Source: CAD feature listing. Evaluate the final solid. Frame: model axes, mm. Face numbers are marked on the shaded views. A direction names the side the tool comes from. Give positions to 0.01 mm unless a question says otherwise; leave off trailing zeros. Order: outer loops, then holes, each group sorted by start corner. A loop starts at its lowest first (then second) coordinate and runs counter-clockwise, first axis right, second up.
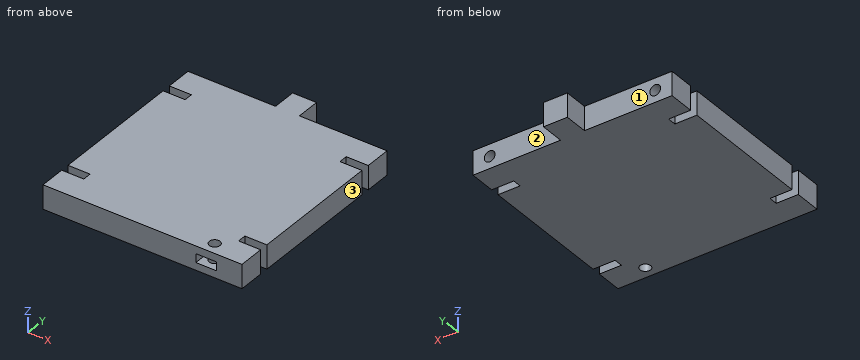
Autodesk Inventor part; units mm, degrees
ref_plane "YZ Plane" through (0, 0, 0) normal (1, 0, 0) x (0, 1, 0)
ref_plane "XZ Plane" through (0, 0, 0) normal (0, 1, 0) x (-1, 0, 0)
ref_plane "XY Plane" through (0, 0, 0) normal (0, 0, 1) x (1, 0, 0)
sketch "스케치1" plane through (0, 0, 0) normal (0, 0, 1) x (1, 0, 0)
  line L0 (0, 0) -> (50, 0)
  line L1 (50, 0) -> (50, 25)
  line L2 (0, 25) -> (50, 25)
  line L3 (0, 0) -> (0, 25)
  line L4 (8.4, 0) -> (0, 0)
  line L5 (0, 0) -> (0, -16)
  line L6 (50, -16) -> (0, -16)
  line L7 (50, 0) -> (50, -16)
  line L8 (50, 0) -> (41.6, 0)
  line L9 (41.6, 0) -> (41.6, -10)
  line L10 (41.6, -10) -> (8.4, -10)
  line L11 (8.4, 0) -> (8.4, -10)
  line L12 (0, 25) -> (50, 25)
  line L13 (50, 25) -> (50, 35)
  line L14 (50, 35) -> (0, 35)
  line L15 (0, 35) -> (0, 25)
  line L16 (0, -16) -> (50, -16)
  line L17 (50, -16) -> (50, 35)
  line L18 (50, 35) -> (0, 35)
  line L19 (0, 35) -> (0, -16)
  dimension "d0" = 10
extrude "돌출1" add sketch "스케치1" along normal blind 6
sketch "스케치2" plane through (0, 0, 6) normal (0, 0, 1) x (1, 0, 0)
  circle A0 centre (41, -13) radius 1.35
  point P0 (0, 0)
extrude "돌출2" cut sketch "스케치2" against normal up to next
sketch "스케치3" plane through (0, 35, 0) normal (0, 1, 0) x (1, 0, 0)
  line L0 (50, 0) -> (0, 0)
  line L1 (28, -6) -> (50, -6)
  line L2 (39, -6) -> (25, 0)
  line L3 (39, -6) -> (22, -6)
  line L4 (22, -6) -> (22, 0)
  line L5 (22, 0) -> (39, 0)
  line L6 (39, 0) -> (39, -6)
  line L7 (39, 0) -> (28, 0)
  line L8 (28, 0) -> (28, -6)
  line L9 (28, -6) -> (39, -6)
  line L10 (39, -6) -> (39, 0)
  point P0 (22, -6)
extrude "돌출3" add sketch "스케치3" along normal blind 6 contours L8 L2 L0 | L2 L8 L3 L4 L0
sketch "스케치4" plane through (50, 35, 6) normal (0, 1, 0) x (1, 0, 0)
  circle A0 centre (-4.2, 79) radius 1.35
  circle A1 centre (-4.2, 3) radius 1.35
  circle A2 centre (-45.8, 79) radius 1.35
  circle A3 centre (-45.8, 3) radius 1.35
  circle A4 centre (-4.2, 71.8) radius 1.6
  circle A5 centre (-45.8, 71.8) radius 1.6
  circle A6 centre (-4.2, 10.2) radius 1.6
  circle A7 centre (-45.8, 10.2) radius 1.6
  line L0 (-50, 0) -> (-28, 0)
  line L1 (-28, 0) -> (-28, 6)
  line L2 (-28, 6) -> (-22, 6)
  line L3 (-22, 6) -> (-22, 0)
  line L4 (-22, 0) -> (0, 0)
  line L5 (0, 0) -> (0, 82)
  line L6 (0, 82) -> (-50, 82)
  line L7 (-50, 82) -> (-50, 0)
  point P0 (-50, 6)
extrude "돌출4" cut sketch "스케치4" against normal blind 6 contours A1 | A3
sketch "스케치6" plane through (0, 0, 6) normal (0, 0, 1) x (1, 0, 0)
  line L0 (47.05, 26.225) -> (47.05, 40.9)
  line L1 (47.05, 31.225) -> (47.05, 40.9)
  line L2 (47.05, 26.225) -> (49.65, 26.225)
  line L3 (50, -16) -> (50, 35)
  line L4 (47.05, 26.225) -> (44.45, 26.225)
  line L5 (44.45, 26.225) -> (44.45, 28.425)
  line L6 (44.45, 28.425) -> (49.65, 28.425)
  line L7 (49.65, 28.425) -> (49.65, 26.225)
  line L8 (28, 41) -> (22, 41)
  line L9 (25, 41) -> (25, 38)
  line L10 (2.95, 26.225) -> (0.35, 26.225)
  line L11 (2.95, 26.225) -> (5.55, 26.225)
  line L12 (5.55, 26.225) -> (5.55, 28.425)
  line L13 (5.55, 28.425) -> (0.35, 28.425)
  line L14 (0.35, 28.425) -> (0.35, 26.225)
  line L15 (0, 35) -> (0, -16)
  line L16 (0.35, 26.225) -> (0, 26.225)
  line L17 (0, 26.225) -> (0, 28.425)
  line L18 (0, 28.425) -> (0.35, 28.425)
  line L19 (0.35, 28.425) -> (0.35, 26.225)
  line L20 (49.65, 28.425) -> (50, 28.425)
  line L21 (50, 28.425) -> (50, 26.225)
  line L22 (50, 26.225) -> (49.65, 26.225)
  line L23 (49.65, 26.225) -> (49.65, 28.425)
  line L24 (0, 9.5) -> (2.95, 9.5)
  line L25 (47.05, -7.225) -> (49.65, -7.225)
  line L26 (47.05, -7.225) -> (44.45, -7.225)
  line L27 (44.45, -7.225) -> (44.45, -9.425)
  line L28 (44.45, -9.425) -> (49.65, -9.425)
  line L29 (49.65, -9.425) -> (49.65, -7.225)
  line L30 (2.95, -7.225) -> (0.35, -7.225)
  line L31 (2.95, -7.225) -> (5.55, -7.225)
  line L32 (5.55, -7.225) -> (5.55, -9.425)
  line L33 (5.55, -9.425) -> (0.35, -9.425)
  line L34 (0.35, -9.425) -> (0.35, -7.225)
  line L35 (0.35, -7.225) -> (0, -7.225)
  line L36 (0, -7.225) -> (0, -9.425)
  line L37 (0, -9.425) -> (0.35, -9.425)
  line L38 (0.35, -9.425) -> (0.35, -7.225)
  line L39 (49.65, -9.425) -> (50, -9.425)
  line L40 (50, -9.425) -> (50, -7.225)
  line L41 (50, -7.225) -> (49.65, -7.225)
  line L42 (49.65, -7.225) -> (49.65, -9.425)
  point P0 (0, 0)
  point P1 (47.05, -12.225)
  point P2 (0, -7.225)
  point P3 (0, 26.225)
  dimension "d11" = 2.6
  dimension "d12" = 2.6
  dimension "d13" = 2.2
extrude "돌출6" cut sketch "스케치6" against normal up to next
sketch "스케치7" plane through (0, -16, 0) normal (0, -1, 0) x (1, 0, 0)
  line L0 (42.25, -2.775) -> (42.25, 11.9)
  line L1 (39.75, -2.775) -> (39.75, 11.9)
  line L2 (42.25, -2.775) -> (39.75, -2.775)
  line L3 (41, -2.775) -> (41, 6)
  line L4 (41, 0) -> (41, 6)
  line L5 (41, 3) -> (43.6, 3)
  line L6 (41, 3) -> (38.4, 3)
  line L7 (43.6, 3) -> (38.4, 3)
  line L8 (38.4, 3) -> (38.4, 1.9)
  line L9 (38.4, 1.9) -> (43.6, 1.9)
  line L10 (43.6, 1.9) -> (43.6, 3)
  line L11 (38.4, 3) -> (38.4, 4.1)
  line L12 (38.4, 4.1) -> (43.6, 4.1)
  line L13 (43.6, 4.1) -> (43.6, 3)
  point P0 (0, 0)
  dimension "d16" = 2.6
  dimension "d17" = 2.6
  dimension "d18" = 1.1
extrude "돌출7" cut sketch "스케치7" against normal blind 6 contours L9 L3 L5 L0 | L0 L5 L10 L9 | L5 L3 L12 L0 | L0 L12 L13 L5 | L9 L1 L6 L3 | L6 L1 L12 L3 | L9 L8 L6 L1 | L6 L11 L12 L1
properties part number "head_side"
1) Section query B-B, the plane y = -13. Return the cut outline in (x, z), and give its area (3 significant figures).
Report:
outline: (0, 0) - (39.65, 0) - (39.65, 1.9) - (38.4, 1.9) - (38.4, 4.1) - (39.65, 4.1) - (39.65, 6) - (0, 6) - close; (42.35, 0) - (50, 0) - (50, 6) - (42.35, 6) - (42.35, 4.1) - (43.6, 4.1) - (43.6, 1.9) - (42.35, 1.9) - close
area: 278 mm2
2) Section query A-A, the plane x = 45.8. Return the cut outline in (y, z) (3 decimals).
Report:
outline: (-16, 0) - (-9.425, 0) - (-9.425, 6) - (-16, 6) - close; (-7.225, 0) - (26.225, 0) - (26.225, 6) - (-7.225, 6) - close; (28.425, 0) - (35, 0) - (35, 1.65) - (29, 1.65) - (29, 4.35) - (35, 4.35) - (35, 6) - (28.425, 6) - close
3) Reachability of the marked faces 1, 2 and 3 from +Z, -Z, +X, -X, +Y, -Y: full face, straight path, thin tool, end or side. Return the list, or none.
Report:
face 1: +Z, -Z, -X, +Y
face 2: +Z, -Z, +X, +Y
face 3: +Z, -Z, +X, +Y, -Y
4) Section query C-C, the plane z = 5. Return the cut outline in (x, y) (3 decimals), and give its area (3 significant figures).
Report:
outline: (0, -16) - (50, -16) - (50, -9.425) - (44.45, -9.425) - (44.45, -7.225) - (50, -7.225) - (50, 26.225) - (44.45, 26.225) - (44.45, 28.425) - (50, 28.425) - (50, 35) - (28, 35) - (28, 41) - (22, 41) - (22, 35) - (0, 35) - (0, 28.425) - (5.55, 28.425) - (5.55, 26.225) - (0, 26.225) - (0, -7.225) - (5.55, -7.225) - (5.55, -9.425) - (0, -9.425) - close; hole circle Ø2.7 at (41, -13)
area: 2,530 mm2
5) Section query D-D, the plane x = 6.5. Return the cut outline in (y, z), and give its area (3 significant figures).
Report:
outline: (-16, 0) - (35, 0) - (35, 6) - (-16, 6) - close
area: 306 mm2
6) Pin query (flat end, axial travel): pin 1 (2 mm diameter, centred on x = 41, y = -13, fed in from -Z); pin 2 (1.8 mm diameter, centred on y = 38, z = 3.5, fed in from -X); pin 3 (3 mm diameter, centred on x = 11.5, z = 3, fed in from +Y); pin 4 (0.7 mm diameter, centred on y = -9, z = 1.5, fed in from -X). Return the tip coordinate at first contact, or that it passes through.
Report:
pin 1: passes through
pin 2: stops at x = 22
pin 3: stops at y = 35
pin 4: stops at x = 5.55
7) Material intervals for L1, parallel to X at y = 30.3, z = 3; L2, parallel to Y at x = 45, z = 3.9 (3 decimals); L3, parallel to Z at x = 4.2, y = 32.1, sorted ascending.
Report:
L1: x = 0 to 2.85, 5.55 to 44.45, 47.15 to 50
L2: y = -16 to -9.425, -7.225 to 26.225, 28.425 to 29
L3: z = 0 to 1.65, 4.35 to 6
